For this review, take the finished solid that the model builds, in its own axes (mm). A direction names the side the tool comes from. Round coordinates to 2 decimals unless told otherwise and drop trailing zeros. Loops run counter-clockwise (first coordinate to the right, second up) from the corner with the lowest first, then second, coordinate; pieces in that order, holes last.
1. Consider section A-A on x = 45. State the section outline as (y, z) points, then the cut area to 3 significant figures.
2. Clearance check with flat-ended pins moving along their axes: pin 1 Ø3 at (x, y) = (47, -6.5) entering from -Z; pin 2 Ø1.5 at (x, z) = (12, -9) entering from -Y; pin 3 Ø3 at (x, y) = (47, -10) entering from +Z. State where each tip first meets the part, or that it passes through.
3. Consider section C-C on z = 22. State the section outline as (x, y) points, then the cut area to 3 significant figures.
4. To check wall thickness, follow line 1 along Y through (x, z) = (45, 1.5); line 2 along X through (y, z) = (-9, 1.5); line 3 along X through (y, z) = (-11.5, -4.5). State the ranges of each line that lie inside material, in increasing order.
5. Consider section B-B on y = -7.5. State the section outline as (x, z) points, then the cut area to 3 significant figures.
6. Tool access review of faces 1 (the flat face through (40, -7, 0)), 2 (the flat face through (44, -5, 5.013)), 3 (the cylindrical face through (-42.69, -8.46, 0.08)), 4 (the flat face through (44, -5, -4.987)): name each direction out of +Z, -Z, +X, -X, +Y, -Y from which nothing blocks a thin tool from reaching the whole face with its end or side.
7. Draft analysis for pull direction X (two halves, no side actions). For faces 5 (the cylindrical face through (47.31, -8.46, 0.08)), 6 (the flat face through (50, -2, 1)), 7 (the flat face through (-46, -5, 5.013)), state which applies: released by +X, released by -X, zero draft, split by the parting line, or undercut.
from build123d import *

# Parameters (mm, degrees)
SKETCH1_W           = 100
SKETCH1_H           = 80
BOSS_EXTRUDE1_DEPTH = 2.5
SKETCH3_W           = 10
SKETCH3_H           = 10
BOSS_EXTRUDE2_DEPTH = 10
SKETCH6_R           = 2.5
CUT_EXTRUDE2_DEPTH  = 10


with BuildPart() as part:
    # Sketch1 → Boss-Extrude1 (new, symmetric)
    with BuildSketch(Plane(origin=(0, 0, 0), x_dir=(1, 0, 0), z_dir=(0, 1, 0))):
        Rectangle(SKETCH1_W, SKETCH1_H)
    extrude(amount=BOSS_EXTRUDE1_DEPTH, both=True)

    # Sketch3 → Boss-Extrude2 (add)
    with BuildSketch(Plane.XZ.offset(2.5)):
        with Locations((-45, 0.013089728)):
            Rectangle(SKETCH3_W, SKETCH3_H)
        with Locations((45, 0.013089728)):
            Rectangle(SKETCH3_W, SKETCH3_H)
    extrude(amount=BOSS_EXTRUDE2_DEPTH)

    # Sketch6 → Cut-Extrude2 (cut)
    with BuildSketch(Plane.XY.offset(5.013089728)):
        with Locations((-45, -7.5)):
            Circle(SKETCH6_R)
        with Locations((45, -7.5)):
            Circle(SKETCH6_R)
    extrude(amount=-CUT_EXTRUDE2_DEPTH, mode=Mode.SUBTRACT)


solid = part.part
Resolved:
1. outline: (-12.5, -4.99) - (-10, -4.99) - (-10, 5.01) - (-12.5, 5.01) - close; (-5, -4.99) - (-2.5, -4.99) - (-2.5, -40) - (2.5, -40) - (2.5, 40) - (-2.5, 40) - (-2.5, 5.01) - (-5, 5.01) - close
1. area: 450 mm2
2. pin 1: stops at z = -4.99
2. pin 2: stops at y = -2.5
2. pin 3: stops at z = 5.01
3. outline: (-50, -2.5) - (50, -2.5) - (50, 2.5) - (-50, 2.5) - close
3. area: 500 mm2
4. line 1: y = -12.5 to -10, -5 to 2.5
4. line 2: x = -50 to -47, -43 to -40, 40 to 43, 47 to 50
4. line 3: x = -50 to -40, 40 to 50
5. outline: (-50, -4.99) - (-47.5, -4.99) - (-47.5, 5.01) - (-50, 5.01) - close; (-42.5, -4.99) - (-40, -4.99) - (-40, 5.01) - (-42.5, 5.01) - close; (40, -4.99) - (42.5, -4.99) - (42.5, 5.01) - (40, 5.01) - close; (47.5, -4.99) - (50, -4.99) - (50, 5.01) - (47.5, 5.01) - close
5. area: 100 mm2
6. face 1: +Z, -Z, -Y
6. face 2: +Z, +X, -X, -Y
6. face 3: +Z, -Z
6. face 4: -Z, +X, -X, -Y
7. face 5: undercut
7. face 6: released by +X
7. face 7: zero draft
